Work out the finished part from the listing and answer in its coordinate system (mm). Round coordinates to 2 decimals unless told otherwise and drop trailing zeros. Loops run counter-clockwise (first coordinate to the right, second up) from the corner with the lowest first, then second, coordinate; pieces in that order, holes last.
```python
from build123d import *

# Parameters (mm, degrees)
F0_R     = 3
F1_DEPTH = 3
F2_SIZE  = 0.5
F3_SIZE  = 2


with BuildPart() as f1:
    # F0 (on Front) → F1 (new body)
    with BuildSketch(Plane.XZ):
        with BuildLine():
            ThreePointArc((5, 0), (15, -10), (25, 0))
            ThreePointArc((25, 0), (0, 25), (-25, 0))
            ThreePointArc((-25, 0), (-23.625052, -5.060482), (-19.878305, -8.729384))
            Line((-19.878305, -8.729384), (-19.105368, -9.351182))
            ThreePointArc((-19.105368, -9.351182), (-13.00964, -15.035608), (-10.128077, -22.856554))
            Line((-10.128077, -22.856554), (-5.949082, -54.729208))
            ThreePointArc((-5.949082, -54.729208), (-3.957266, -58.459186), (0, -59.949192))
            Line((0, -59.949192), (0, -5))
            ThreePointArc((0, -5), (-3.535534, 3.535534), (5, 0))
        make_face()
        with Locations((-15, 0)):
            Circle(F0_R, mode=Mode.SUBTRACT)
        with Locations((15, 0)):
            Circle(F0_R, mode=Mode.SUBTRACT)
    extrude(amount=F1_DEPTH)

    # F2
    f2_edges = [f1.edges().sort_by_distance(p)[0] for p in [
        (-18, -3, 0),
        (12, -3, 0),
    ]]
    chamfer(f2_edges, length=F2_SIZE)

    # F3
    f3_edges = [f1.edges().sort_by_distance(p)[0] for p in [
        (0, -3, -32.474596),
    ]]
    chamfer(f3_edges, length=F3_SIZE)


solid = f1.part
```
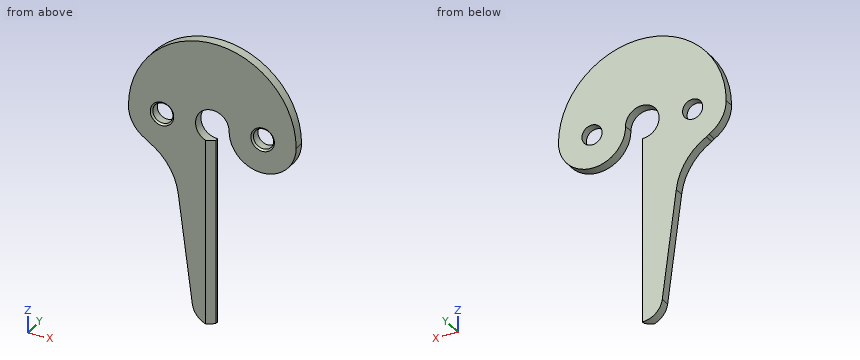
1. Find section A-A (x = 15). Write down the section's boundary in (y, z), then the cut area to 4 significant figures.
Answer key:
outline: (-3, -10) - (0, -10) - (0, -3) - (-2.5, -3) - (-3, -3.5) - close; (-3, 3.5) - (-2.5, 3) - (0, 3) - (0, 20) - (-3, 20) - close
area: 71.75 mm2
2. Given pin 1 (1.5 mm diameter, centred on x = 12.5, y = -1, fed in from -Z); pin 2 (9 mm diameter, centred on x = 0, z = 0, fed in from -Y); pin 3 (0.5 mm diameter, centred on y = -0.5, z = -30.5, fed in from +X), each flat-ended and moving along its own axis, determine where each tip first touches the part or whether it passes through.
Answer key:
pin 1: stops at z = -9.85
pin 2: passes through
pin 3: stops at x = 0
3. Find section C-C (z = 7). Write down the section's boundary in (x, y), then the cut area to 3 significant figures.
Answer key:
outline: (-24, -3) - (24, -3) - (24, 0) - (-24, 0) - close
area: 144 mm2
4. Consider probe 1 along Y at (x, z) = (-1.5, -13.5); probe 2 along Z at (x, y) = (17.5, -0.6); probe 3 along Z at (x, y) = (0, -1.65). Determine where each line is inside the solid, lowest interval first.
Answer key:
probe 1: y = -2.5 to 0
probe 2: z = -9.68 to -1.66, 1.66 to 17.85
probe 3: z = 5 to 25
5. Find section B-B (y = -1.75). Write down the section's boundary in (x, z), then the cut area to 3 significant figures.
Answer key:
outline: (-25, 0) arc R10 ccw to (-19.88, -8.73) - (-19.11, -9.35) arc R18 cw to (-10.13, -22.86) - (-5.95, -54.73) arc R6 ccw to (-0.75, -59.9) - (-0.75, -4.94) arc R5 cw (long way) to (5, 0) arc R10 ccw to (25, 0) arc R25 ccw to start; hole circle Ø6 at (-15, 0); hole circle Ø6 at (15, 0)
area: 1,660 mm2
6. Find section D-D (z = -2). Give the number of separate pieces and of enclosed holes in the cut face, then the cut area to 3 significant figures.
Answer key:
separate pieces: 4
enclosed holes: 0
area: 92.0 mm2
